```python
from build123d import *

# Parameters (mm, degrees)
SKETCH1_W                    = 1570
SKETCH1_H                    = 40
BASE_FLANGE1_DEPTH           = 4
EDGE_FLANGE1_STRIP_W         = 28
EDGE_FLANGE1_STRIP_H         = 4
EDGE_FLANGE1_STRIP_CUT_DEPTH = 1570
EDGE_FLANGE1_DEPTH           = 1570
SKETCH9_W                    = 35
SKETCH9_H                    = 6
CUT_EXTRUDE1_DEPTH           = 10
CUT_EXTRUDE2_DEPTH           = 10
LPATTERN1_COUNT              = 11
LPATTERN1_PITCH              = 150


# Sheet-metal steps are written as plain solids
with BuildPart() as part:
    # Sketch1 → Base-Flange1 (new body)
    with BuildSketch(Plane(origin=(0, 0, 0), x_dir=(1, 0, 0), z_dir=(0, 1, 0))):
        with Locations((-479.623655914, 20)):
            Rectangle(SKETCH1_W, SKETCH1_H)
    extrude(amount=-BASE_FLANGE1_DEPTH)

    # Edge-Flange1 strip (across the edge) → Edge-Flange1 strip cut (cut)
    with BuildSketch(Plane(origin=(305.376344086, 0, -40), x_dir=(0, 0, 1), z_dir=(-1, 0, 0))):
        with Locations((-4, -2)):
            Rectangle(EDGE_FLANGE1_STRIP_W, EDGE_FLANGE1_STRIP_H)
    extrude(amount=EDGE_FLANGE1_STRIP_CUT_DEPTH, mode=Mode.SUBTRACT)

    # Edge-Flange1 section (across the edge) → Edge-Flange1 (add)
    with BuildSketch(Plane(origin=(305.376344086, 0, -40), x_dir=(0, 0, 1), z_dir=(-1, 0, 0))):
        with BuildLine():
            Line((0, 6), (0, 36))
            Line((0, 36), (4, 36))
            Line((4, 36), (4, 6))
            ThreePointArc((4, 6), (5.757359313, 1.757359313), (10, 0))
            Line((10, 0), (10, -4))
            ThreePointArc((10, -4), (2.928932188, -1.071067812), (0, 6))
        make_face()
    extrude(amount=EDGE_FLANGE1_DEPTH)

    # Sketch9 → Cut-Extrude1 (cut)
    with BuildSketch(Plane.XY.offset(-36)):
        with Locations((287.876344086, 33)):
            Rectangle(SKETCH9_W, SKETCH9_H)
        with Locations((-1247.123655914, 33)):
            Rectangle(SKETCH9_W, SKETCH9_H)
    extrude(amount=-CUT_EXTRUDE1_DEPTH, mode=Mode.SUBTRACT)

    # Sketch10 → Cut-Extrude2 (cut)
    with BuildSketch(Plane.XY.offset(-36)):
        with BuildLine():
            Line((273.376344086, 11.5), (267.376344086, 11.5))
            ThreePointArc((267.376344086, 11.5), (262.876344086, 16), (267.376344086, 20.5))
            Line((267.376344086, 20.5), (273.376344086, 20.5))
            ThreePointArc((273.376344086, 20.5), (277.876344086, 16), (273.376344086, 11.5))
        make_face()
    cut_extrude2 = extrude(amount=-CUT_EXTRUDE2_DEPTH, mode=Mode.SUBTRACT)

    # LPattern1: Cut-Extrude2 ×11
    with Locations(*[(-i * LPATTERN1_PITCH, 0, 0) for i in range(1, LPATTERN1_COUNT)]):
        add(cut_extrude2, mode=Mode.SUBTRACT)


solid = part.part
```
Source: CAD feature listing. Evaluate the final solid. Frame: model axes, mm. A direction names the side the tool comes from. Round coordinates to 2 decimals unless told otherwise and drop trailing zeros. Loops run counter-clockwise (first coordinate to the right, second up) from the corner with the lowest first, then second, coordinate; pieces in that order, holes last. Notation, with made-up numbers: M 8,7.25 L 61,7.25 A12 ccw 61,13.25 Z; hole C 5.5,86.5 d6. An arc over 180 degrees is marked long. Use a Markdown table: item, result. Add a question column.
1. Cut plane A-A, the plane x = -566. Output: boundary loops of the cut face in (y, z).
2. Ray query, line 1 along Y through (x, z) = (-969, -20); line 2 along Z through (x, y) = (17.5, 15); line 3 along Z through (x, y) = (149, 4.5). Return the intervals inside material, ascending. Write a range as [from, to].
3. Contact query for flat-ended pins moving along their axis: pin 1 (4.5 mm diameter, centred on x = -929.5, z = -39, fed in from -Y); pin 2 (4.5 mm diameter, centred on x = -1229.5, z = -38, fed in from -Y); pin 3 (4 mm diameter, centred on x = -342.5, z = -17, fed in from +Y). Output: stop coordinate, or through.
4. Set-up query: faces 1 (the flat face through (-469, 21, -40)), 2 (the flat face through (-469, 21, -36)). Return all of +Z, -Z, +X, -X, +Y, -Y with unobstructed straight access to the full face (end or side cutting, diameter ignored); none if empty.
5. Cut plane B-B, the plane z = -19. Output: boundary loops of the cut face in (x, y), and give its area (3 significant figures).
Solution:
| question | item | result |
|---|---|---|
| 1 | outline | M -4,-30 A10 ccw 6,-40 L 36,-40 L 36,-36 L 6,-36 A6 cw 0,-30 L 0,0 L -4,0 Z |
| 2 | line 1 | y = [-4, 0] |
| 2 | line 2 | z = [-40, -36] |
| 2 | line 3 | z = [-39.89, -35.81] |
| 3 | pin 1 | stops at y = -1.38 |
| 3 | pin 2 | stops at y = -2.18 |
| 3 | pin 3 | stops at y = 0 |
| 4 | face 1 | -Z, +X, -X, +Y, -Y |
| 4 | face 2 | +Z, +X, -X, +Y |
| 5 | outline | M -1264.62,-4 L 305.38,-4 L 305.38,0 L -1264.62,0 Z |
| 5 | area | 6,280 mm2 |
